Verification items for the finished model (mm, model axes). Face numbers are marked on the shaded views. A direction names the side the tool comes from. Round coordinates to 2 decimals unless told otherwise and drop trailing zeros. Write each loop counter-clockwise with the first axis right and the second up, starting at its lowest first coordinate (ties: lowest second). Pieces come first, ordered by that corner, then holes. Notation, with made-up numbers: (37, -7.75) - (88, -7.75) arc R24 ccw to (88, 16.25) - close; hole circle Ø3 at (82.5, 73). An arc over 180 degrees is marked (long way). Answer as a JSON object with one key per item and string values. Group by question number.
1) Set-up check for the marked faces 1 and 2: record each of +Z, -Z, +X, -X, +Y, -Y from which the full face is reachable in a straight line by a thin tool's end or side.
2) Section check B-B (z = 38.1). Enter the section's corners in (x, y).
3) Section check A-A (z = 63.5). Enter the section's corners in (x, y).
4) Section check C-C (y = 51). Enter the section's corners in (x, z), then the cut area to 3 significant figures.
5) Go/stop test with flat-tipped pins: pin 1 Ø22 at (y, z) = (37.5, 53.5) entering from +X; pin 2 Ø4 at (y, z) = (26.21, 38.1) entering from -X; pin 3 Ø7.5 at (x, z) = (7.33, 12.7) entering from -Y; pin 4 Ø24 at (x, z) = (-8, 57) entering from +Y. Record where each tip stops, or that it passes through.
6) Thickness scan on line 1 (Y direction, x = -29, z = 38.1); line 2 (X direction, y = -9.9, z = 12.7); line 3 (X direction, y = -9, z = 12). Record the ranges inside material, lowest first.
7) Section check D-D (z = 17). Enter the section's corners in (x, y).
Autodesk Inventor part; units mm, degrees
ref_plane "YZ Plane" through (0, 0, 0) normal (1, 0, 0) x (0, 1, 0)
ref_plane "XZ Plane" through (0, 0, 0) normal (0, 1, 0) x (-1, 0, 0)
ref_plane "XY Plane" through (0, 0, 0) normal (0, 0, 1) x (1, 0, 0)
sketch "Sketch1" plane through (0, 0, 0) normal (0, 0, 1) x (1, 0, 0)
  line L0 (-30.7726, 64.3138) -> (-30.7726, -11.8862)
  line L1 (-30.7726, -11.8862) -> (20.0274, -11.8862)
  line L2 (20.0274, -11.8862) -> (20.0274, -8.8382)
  line L3 (20.0274, -8.8382) -> (-27.7246, -8.8382)
  line L4 (-27.7246, -8.8382) -> (-27.7246, 64.3138)
  line L5 (-27.7246, 64.3138) -> (-30.7726, 64.3138)
  point P0 (0, 0)
  dimension "d0" = 3.048
  dimension "d1" = 3.048
  dimension "d2" = 76.2
  dimension "d3" = 50.8
extrude "Extrusion1" add sketch "Sketch1" along normal blind 76.2
sketch "Sketch2" plane through (-30.7726, -11.8862, 0) normal (-1, 0, 0) x (0, 0, 1)
  line L0 (0, 76.2) -> (0, 0)
  line L1 (0, 0) -> (76.2, 0)
  point P0 (0, 11.8862)
  point P1 (38.1, 57.15)
  point P2 (38.1, 38.1)
  point P3 (38.1, 19.05)
  dimension "d6" = 19.05
  dimension "d7" = 38.1
  dimension "d8" = 57.15
  dimension "d9" = 38.1
  dimension "d10" = 38.1
  dimension "d11" = 38.1
hole "Hole1" at (-30.7726, 45.2638, 38.1) at (-30.7726, 26.2138, 38.1) at (-30.7726, 7.1638, 38.1) direction (1, 0, 0) diameter 6.35 depth 25.4 tip angle 118
thread "Thread1"
thread "Thread2"
thread "Thread3"
sketch "Sketch3" plane through (-27.7246, -8.8382, 0) normal (0, 1, 0) x (1, 0, 0)
  line L0 (0, -76.2) -> (47.752, -76.2)
  line L1 (47.752, 0) -> (47.752, -76.2)
  line L2 (47.752, 0) -> (0, 0)
  point P0 (27.7246, 0)
  point P1 (9.652, -63.5)
  point P2 (9.652, -12.7)
  point P3 (35.052, -12.7)
  point P4 (35.052, -63.5)
  dimension "d30" = 12.7
  dimension "d31" = 12.7
  dimension "d32" = 12.7
  dimension "d33" = 12.7
  dimension "d34" = 12.7
  dimension "d35" = 38.1
  dimension "d36" = 12.7
  dimension "d37" = 38.1
hole "Hole2" at (-18.0726, -8.8382, 63.5) at (-18.0726, -8.8382, 12.7) at (7.3274, -8.8382, 12.7) at (7.3274, -8.8382, 63.5) direction (0, -1, 0) diameter 6.35 depth 25.4 tip angle 118
thread "Thread4"
thread "Thread5"
thread "Thread6"
thread "Thread7"
properties part number "curveBracket"
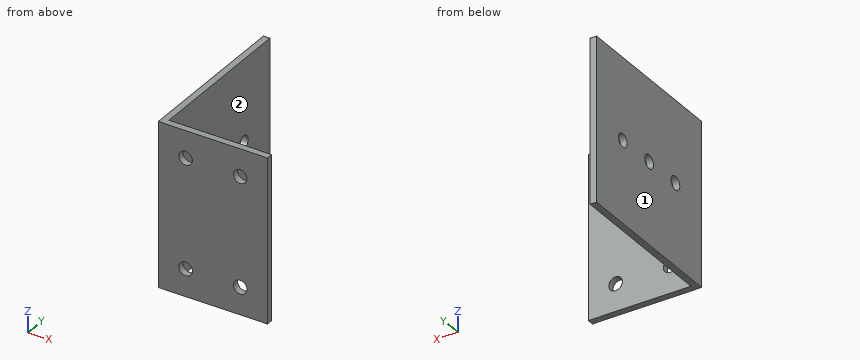
Returned:
{
 "1": {"face 1": "+Z, -Z, -X, +Y, -Y", "face 2": "+Z, -Z, +X, +Y"},
 "2": {"outline": "(-30.77, -11.89) - (20.03, -11.89) - (20.03, -8.84) - (-27.72, -8.84) - (-27.72, 3.99) - (-30.77, 3.99) - close; (-30.77, 10.34) - (-27.72, 10.34) - (-27.72, 23.04) - (-30.77, 23.04) - close; (-30.77, 29.39) - (-27.72, 29.39) - (-27.72, 42.09) - (-30.77, 42.09) - close; (-30.77, 48.44) - (-27.72, 48.44) - (-27.72, 64.31) - (-30.77, 64.31) - close"},
 "3": {"outline": "(-30.77, -11.89) - (-21.25, -11.89) - (-21.25, -8.84) - (-27.72, -8.84) - (-27.72, 64.31) - (-30.77, 64.31) - close; (-14.9, -11.89) - (4.15, -11.89) - (4.15, -8.84) - (-14.9, -8.84) - close; (10.5, -11.89) - (20.03, -11.89) - (20.03, -8.84) - (10.5, -8.84) - close"},
 "4": {"outline": "(-30.77, 0) - (-27.72, 0) - (-27.72, 76.2) - (-30.77, 76.2) - close", "area": "232 mm2"},
 "5": {"pin 1": "x = -27.72", "pin 2": "through", "pin 3": "y = -11.89", "pin 4": "y = -8.84"},
 "6": {"line 1": "-11.89 to 3.99, 10.34 to 23.04, 29.39 to 42.09, 48.44 to 64.31", "line 2": "-30.77 to -21.25, -14.9 to 4.15, 10.5 to 20.03", "line 3": "-30.77 to -21.17, -14.98 to 4.23, 10.42 to 20.03"},
 "7": {"outline": "(-30.77, -11.89) - (20.03, -11.89) - (20.03, -8.84) - (-27.72, -8.84) - (-27.72, 64.31) - (-30.77, 64.31) - close"}
}
